Work out the finished part from the listing and answer in its coordinate system (mm). A direction names the side the tool comes from. Give positions to 0.01 mm unless a question says otherwise; leave off trailing zeros. Write each loop counter-clockwise with the first axis right and the second up, starting at its lowest first coordinate (ties: lowest second). Pieces come first, ordered by that corner, then holes. Notation, with made-up numbers: (-16.5, 54) -> (14.5, 54) arc R14 cw to (14.5, 65) -> close; hole circle Ø11 at (8.5, 53). An arc over 180 degrees is marked (long way). Use a Markdown table: item, result. Add a question column.
Q1. Section C-C, the plane z = 14.25 is taken. Give the vertices of the cut face in (x, y), plus the area to 3 significant figures.
Q2. For faces 4 (the face through (78.015, 16.184, 4.437)), 5 (the face through (88.15, -10.53, 5.96)), 6 (the face through (167, -9, 7)), 7 (the face through (156, 0, 8)), 8 (the face through (56, 0, 0)), determine the directions among +Z, -Z, +X, -X, +Y, -Y from which every point of the face is accessible in a straight line to the end or side of a thin tool.
Q3. Each of these flat-tipped pins is pushed along its axis until it touches: pin 1 Ø11 at (x, y) = (163, 1) entering from -Z; pin 2 Ø8 at (x, y) = (1, -0.5) entering from -Z; pin 3 Ø21 at (x, y) = (108.5, -4.5) entering from +Z; pin 4 Ø4 at (y, z) = (-13, 4) entering from +X. Where does it stop, or does it pass through?
Q4. Section B-B, the plane x = 116 is taken. Give the vertices of the cut face in (y, z), plus the area to 3 significant figures.
Q5. Section D-D, the plane x = 5 is taken. Give the vertices of the cut face in (y, z).
Q6. For a pull along Y with two mould halves and no side action, classify faces 1 (the face through (80, 13, 9)), 2 (the face through (75.861, -16.316, 4.437)), 3 (the face through (154, 0, 3)) as pulls with the +Y half, pulls with the -Y half, needs draft (parallel to the pull), parting line crosses it, or undercut.
Q7. Consider line 1 (Y direction, x = 165, z = 8.15); line 2 (Y direction, x = 165, z = 4.5); line 3 (Z direction, x = 92, y = -8.5). Determine where each line is inside the solid, lowest interval first.
Q8. Section A-A, the plane x = 165 is taken. Give the vertices of the cut face in (y, z).
from build123d import *
from build123d.topology import SkipClean

# Parameters (mm, degrees)
SKETCH6_R           = 9
BOSS_EXTRUDE2_DEPTH = 9
SKETCH6_10_R        = 16
BOSS_EXTRUDE3_DEPTH = 16
CUT_EXTRUDE2_REACH  = 187.915
CUT_EXTRUDE2_START  = 3
SKETCH6_20_R        = 11
CUT_EXTRUDE5_DEPTH  = 7


with BuildPart() as part:
    # Sketch6 → Boss-Extrude2 (new body)
    with BuildSketch(Plane.XY):
        with BuildLine():
            Line((0, -21), (153.875702269, -11.5))
            ThreePointArc((153.875702269, -11.5), (181, 0), (153.875702269, 11.5))
            Line((153.875702269, 11.5), (0, 21))
            ThreePointArc((0, 21), (-21, 0), (0, -21))
        make_face()
        with Locations((165, 0)):
            Circle(SKETCH6_R, mode=Mode.SUBTRACT)
        with BuildLine():
            ThreePointArc((41.185040199, -13.422236438), (40.356373264, -13.49895246), (39.524556783, -13.524556783))
            Line((39.524556783, -13.524556783), (41.185040199, -13.422236438))
        make_face(mode=Mode.SUBTRACT)
        with BuildLine():
            ThreePointArc((39.524556783, 13.524556783), (40.356373264, 13.49895246), (41.185040199, 13.422236438))
            Line((41.185040199, 13.422236438), (39.524556783, 13.524556783))
        make_face(mode=Mode.SUBTRACT)
    extrude(amount=BOSS_EXTRUDE2_DEPTH)

    # Sketch6<10> → Boss-Extrude3 (add)
    with BuildSketch(Plane.XY):
        Circle(SKETCH6_10_R)
    extrude(amount=BOSS_EXTRUDE3_DEPTH)

    # Sketch6<13> → Cut-Extrude2 (cut, up to next)
    with BuildSketch(Plane.XY.offset(CUT_EXTRUDE2_START), mode=Mode.PRIVATE) as cut_extrude2_sk1:
        with BuildLine():
            ThreePointArc((39.524556783, 13.524556783), (29.961250969, 9.563305814), (26, 0))
            Line((26, 0), (144, 0))
            ThreePointArc((144, 0), (141.788053239, 5.34011187), (136.447941368, 7.552058632))
            Line((136.447941368, 7.552058632), (41.185040199, 13.422236438))
            Line((41.185040199, 13.422236438), (39.524556783, 13.524556783))
        make_face()
    cut_extrude2_tool1 = extrude(cut_extrude2_sk1.sketch, amount=CUT_EXTRUDE2_REACH, mode=Mode.PRIVATE) & part.part
    # Sketch6<13> → Cut-Extrude2 (cut, up to next)
    with BuildSketch(Plane.XY.offset(CUT_EXTRUDE2_START), mode=Mode.PRIVATE) as cut_extrude2_sk2:
        with BuildLine():
            Line((144, 0), (26, 0))
            ThreePointArc((26, 0), (29.961250969, -9.563305814), (39.524556783, -13.524556783))
            Line((39.524556783, -13.524556783), (41.185040199, -13.422236438))
            Line((41.185040199, -13.422236438), (136.447941368, -7.552058632))
            ThreePointArc((136.447941368, -7.552058632), (141.788053239, -5.34011187), (144, 0))
        make_face()
    cut_extrude2_tool2 = extrude(cut_extrude2_sk2.sketch, amount=CUT_EXTRUDE2_REACH, mode=Mode.PRIVATE) & part.part
    add(cut_extrude2_tool1.solids().sort_by_distance((79.598695, 5.367714, 3))[0], mode=Mode.SUBTRACT)
    add(cut_extrude2_tool2.solids().sort_by_distance((79.598695, -5.367714, 3))[0], mode=Mode.SUBTRACT)

    # Sketch6<20> → Cut-Extrude5 (cut)
    with SkipClean():  # the faces are left unmerged after this step: merging them gives an invalid solid
        with BuildSketch(Plane.XY):
            with Locations((165, 0)):
                Circle(SKETCH6_20_R)
        extrude(amount=CUT_EXTRUDE5_DEPTH, mode=Mode.SUBTRACT)


solid = part.part
Result set:
| question | item | result |
|---|---|---|
| 1 | outline | circle Ø32 at (0, 0) |
| 1 | area | 804 mm2 |
| 2 | face 4 | +Z, -Z, +Y |
| 2 | face 5 | +Z |
| 2 | face 6 | -Z |
| 2 | face 7 | +Z, -Z |
| 2 | face 8 | -Z, +X, -X, +Y, -Y |
| 3 | pin 1 | passes through |
| 3 | pin 2 | stops at z = 0 |
| 3 | pin 3 | stops at z = 9 |
| 3 | pin 4 | stops at x = 176.62 |
| 4 | outline | (-13.84, 0) -> (13.84, 0) -> (13.84, 9) -> (8.81, 9) -> (8.81, 3) -> (-8.81, 3) -> (-8.81, 9) -> (-13.84, 9) -> close |
| 4 | area | 143 mm2 |
| 5 | outline | (-20.69, 0) -> (20.69, 0) -> (20.69, 9) -> (15.2, 9) -> (15.2, 16) -> (-15.2, 16) -> (-15.2, 9) -> (-20.69, 9) -> close |
| 6 | face 1 | needs draft |
| 6 | face 2 | pulls with the -Y half |
| 6 | face 3 | undercut |
| 7 | line 1 | y = -16 to -9, 9 to 16 |
| 7 | line 2 | y = -16 to -11, 11 to 16 |
| 7 | line 3 | z = 0 to 3 |
| 8 | outline | (-16, 0) -> (-11, 0) -> (-11, 7) -> (-9, 7) -> (-9, 9) -> (-16, 9) -> close; (9, 7) -> (11, 7) -> (11, 0) -> (16, 0) -> (16, 9) -> (9, 9) -> close |
